```python
from build123d import *

# Parameters (mm, degrees)
BOSS_EXTRUDE2_DEPTH             = 6
SKETCH3_W                       = 30
SKETCH3_H                       = 16
BOSS_EXTRUDE3_DEPTH             = 29
CUT_EXTRUDE1_DEPTH              = 16
CUT_EXTRUDE2_DEPTH              = 30
SKETCH6_R                       = 3.5
CUT_EXTRUDE3_DEPTH              = 6
CUT_EXTRUDE4_REACH              = 18
SKETCH7_R                       = 5
BOSS_EXTRUDE4_REACH             = 18
SKETCH8_R                       = 7
SKETCH8_R_2                     = 5
BOSS_EXTRUDE4_DIRECTION_2_DEPTH = 1


with BuildPart() as part:
    # Sketch2 → Boss-Extrude2 (new body)
    with BuildSketch(Plane(origin=(0, 0, 0), x_dir=(1, 0, 0), z_dir=(0, 1, 0))):
        Polygon((-29.5, 8), (-33.5, 4), (-33.5, -4), (-29.5, -8), (29.5, -8), (33.5, -4), (33.5, 4), (29.5, 8), align=None)
    extrude(amount=BOSS_EXTRUDE2_DEPTH)

    # Sketch3 → Boss-Extrude3 (add)
    with BuildSketch(Plane(origin=(0, 6, 0), x_dir=(1, 0, 0), z_dir=(0, 1, 0))):
        Rectangle(SKETCH3_W, SKETCH3_H)
    extrude(amount=BOSS_EXTRUDE3_DEPTH)

    # Sketch4 → Cut-Extrude1 (cut)
    with BuildSketch(Plane.XY.offset(8)):
        with BuildLine():
            ThreePointArc((-15, 20), (-10.606601718, 30.606601718), (0, 35))
            Line((0, 35), (-15, 35))
            Line((-15, 35), (-15, 20))
        make_face()
        with BuildLine():
            Line((15, 20), (15, 35))
            Line((15, 35), (0, 35))
            ThreePointArc((0, 35), (10.606601718, 30.606601718), (15, 20))
        make_face()
    extrude(amount=-CUT_EXTRUDE1_DEPTH, mode=Mode.SUBTRACT)

    # Sketch5 → Cut-Extrude2 (cut)
    with BuildSketch(Plane.ZY.offset(15)):
        Polygon((-6, 35), (-8, 6), (-8, 35), align=None)
        Polygon((8, 6), (6, 35), (8, 35), align=None)
    extrude(amount=-CUT_EXTRUDE2_DEPTH, mode=Mode.SUBTRACT)

    # Sketch6 → Cut-Extrude3 (cut)
    with BuildSketch(Plane.XZ):
        with Locations((-26.5, 0)):
            Circle(SKETCH6_R)
        with Locations((26.5, 0)):
            Circle(SKETCH6_R)
    extrude(amount=-CUT_EXTRUDE3_DEPTH, mode=Mode.SUBTRACT)

    # Cut-Extrude4: up to this face of the body (flat: up to its plane)
    cut_extrude4_end = Plane(part.part.faces().sort_by_distance((0, 19.107869184, 7.096009022))[0])
    # Sketch7 → Cut-Extrude4 (cut, up to the picked face)
    with BuildSketch(Plane(origin=(0, 0, -8), x_dir=(-1, 0, 0), z_dir=(0, 0, -1)), mode=Mode.PRIVATE) as cut_extrude4_sk1:
        with Locations((0, 20)):
            Circle(SKETCH7_R)
    cut_extrude4_tool1 = split(extrude(cut_extrude4_sk1.sketch, amount=-CUT_EXTRUDE4_REACH, mode=Mode.PRIVATE), bisect_by=cut_extrude4_end, keep=Keep.BOTH, mode=Mode.PRIVATE)
    add(cut_extrude4_tool1.solids().sort_by_distance((0, 20, -8))[0], mode=Mode.SUBTRACT)

    # Sketch8 → Boss-Extrude4 (add, up to next)
    with BuildSketch(Plane(origin=(0, 0, -8), x_dir=(-1, 0, 0), z_dir=(0, 0, -1)), mode=Mode.PRIVATE) as boss_extrude4_sk1:
        with Locations((0, 20)):
            Circle(SKETCH8_R)
        with Locations((0, 20)):
            Circle(SKETCH8_R_2, mode=Mode.SUBTRACT)
    boss_extrude4_tool1 = extrude(boss_extrude4_sk1.sketch, amount=-BOSS_EXTRUDE4_REACH, mode=Mode.PRIVATE) - part.part
    add(boss_extrude4_tool1.solids().sort_by_distance((6.80201, 20, -8))[0])

    # Sketch8 → Boss-Extrude4 direction 2 (add)
    with BuildSketch(Plane(origin=(0, 0, -8), x_dir=(-1, 0, 0), z_dir=(0, 0, -1))):
        with Locations((0, 20)):
            Circle(SKETCH8_R)
        with Locations((0, 20)):
            Circle(SKETCH8_R_2, mode=Mode.SUBTRACT)
    extrude(amount=BOSS_EXTRUDE4_DIRECTION_2_DEPTH)


solid = part.part
```
Geometry check sheet. Reference: the model listing, model coordinates, mm. A direction names the side the tool comes from. Round coordinates to 2 decimals unless told otherwise and drop trailing zeros. Order: outer loops, then holes, each group sorted by start corner. A loop starts at its lowest first (then second) coordinate and runs counter-clockwise, first axis right, second up. Notation, with made-up numbers: (29, -17) - (56, -17) arc R19 cw to (56, -2) - close; hole circle Ø3 at (46, 54.5). An arc over 180 degrees is marked (long way). Use a Markdown table: item, result. Add a question column.
1) Thickness scan on line 1 along Z through (x, y) = (26.5, 2.25); line 2 along X through (y, z) = (12, 6); line 3 along Y through (x, z) = (-16, -5). Record the ranges inside material, lowest first.
2) Mould release check, pull along X, two halves, no side actions. Record for faces 4 (the cylindrical face through (-23.16, 2.96, 1.05)), 5 (the flat face through (31.5, 3, -6)), 6 (the flat face through (-31.5, 3, 6)), 7 (the flat face through (-6.88, 17.48, -7.21)): released by +X, released by -X, zero draft, split by the parting line, or undercut.
3) Section check D-D (y = 26). Record the cut outline in (x, z), then the cut area to 3 significant figures.
4) Gauge pin test, flat ends, axial feed: P1, Ø16, axis at x = 0, y = 20, coming from the +Z side; P2, Ø8, axis at x = 4.5, y = 9, coming from the -Z side; P3, Ø5, axis at x = 19.5, z = -4, coming from the +Y side. Record the tip position at first contact, or that the pin passes through.
5) Set-up check for faces 1 (the flat face through (22, 6, 0)), 2 (the cylindrical face through (0.91, 26.94, -7.99)), 3 (the flat face through (0, 3, -8)): record each of +Z, -Z, +X, -X, +Y, -Y from which the full face is reachable in a straight line by a thin tool's end or side.
6) Section check A-A (z = 0). Record the cut outline in (x, y).
7) Section check B-B (x = 26.5). Record the cut outline in (y, z), then the cut area to 3 significant figures.
8) Section check C-C (y = 19). Record the cut outline in (x, z).
Established:
| question | item | result |
|---|---|---|
| 1 | line 1 | -8 to -3.5, 3.5 to 8 |
| 1 | line 2 | -15 to 15 |
| 1 | line 3 | 0 to 6 |
| 2 | face 4 | undercut |
| 2 | face 5 | released by +X |
| 2 | face 6 | released by -X |
| 2 | face 7 | zero draft |
| 3 | outline | (-13.75, -6.62) - (-3.61, -6.62) - (-3.61, -9) - (3.61, -9) - (3.61, -6.62) - (13.75, -6.62) - (13.75, 6.62) - (-13.75, 6.62) - close |
| 3 | area | 381 mm2 |
| 4 | P1 | z = 7.59 |
| 4 | P2 | z = -8 |
| 4 | P3 | y = 6 |
| 5 | face 1 | +Z, -Z, +X, +Y |
| 5 | face 2 | -Z |
| 5 | face 3 | -Z, +X, -X, -Y |
| 6 | outline | (-33.5, 0) - (-30, 0) - (-30, 6) - (-33.5, 6) - close; (-23, 0) - (23, 0) - (23, 6) - (15, 6) - (15, 20) arc R15 ccw to (-15, 20) - (-15, 6) - (-23, 6) - close; (30, 0) - (33.5, 0) - (33.5, 6) - (30, 6) - close; hole circle Ø10 at (0, 20) |
| 7 | outline | (0, -8) - (6, -8) - (6, -3.5) - (0, -3.5) - close; (0, 3.5) - (6, 3.5) - (6, 8) - (0, 8) - close |
| 7 | area | 54.0 mm2 |
| 8 | outline | (-15, -7.1) - (-6.93, -7.1) - (-6.93, -9) - (-4.9, -9) - (-4.9, 7.1) - (-15, 7.1) - close; (4.9, -9) - (6.93, -9) - (6.93, -7.1) - (15, -7.1) - (15, 7.1) - (4.9, 7.1) - close |
